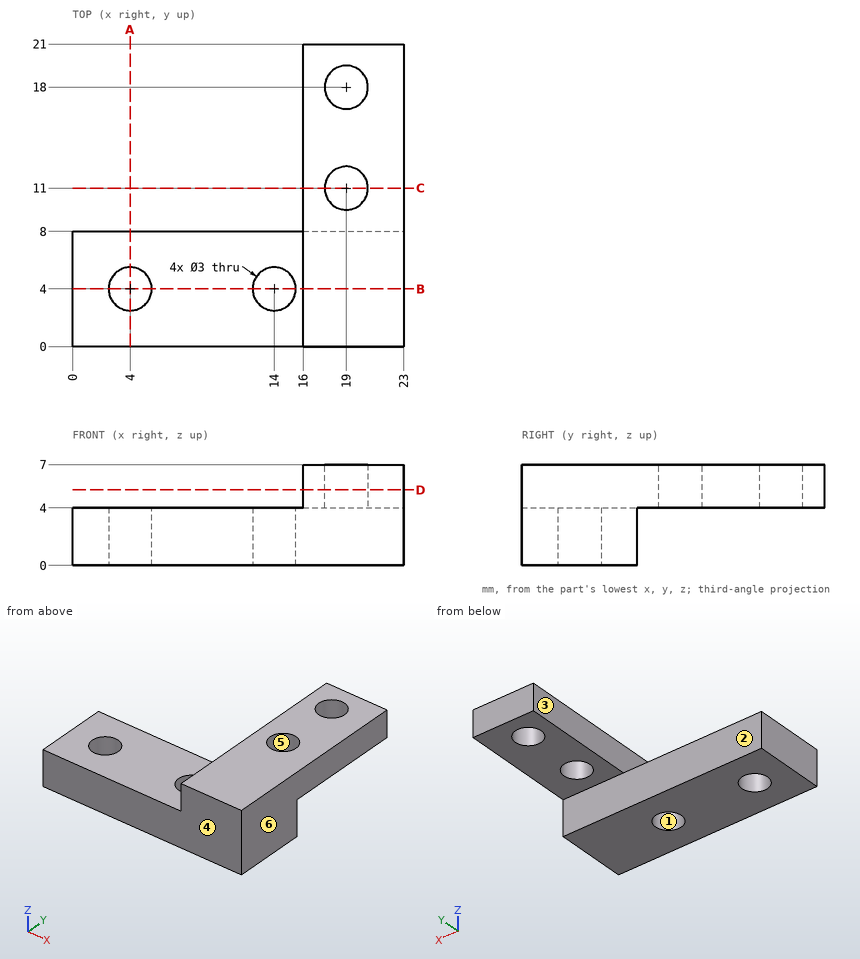
Geometry check sheet. Reference: drawing and pictorial views, mm from the part's lowest x, y, z. A direction names the side the tool comes from. Give positions to 0.01 mm unless a question says otherwise; leave off trailing zeros. Order: outer loops, then holes, each group sorted by start corner. A loop starts at its lowest first (then second) coordinate and runs counter-clockwise, first axis right, second up. Notation, with made-up numbers: (-2, -23) -> (2, -23) arc R34 ccw to (2, 8) -> close; hole circle Ø2 at (72.5, 29.5). An arc over 180 degrees is marked (long way). Use CSV: the item, a comma, the result in double quotes. Start each with the question number.
1) Sectioned sample at D-D, the plane z = 5.25. Record the boundary of the cut face in (x, y).
2) Sectioned sample at A-A, the plane x = 4. Record the boundary of the cut face in (y, z), plus the area to 3 significant figures.
3) Sectioned sample at C-C, the plane y = 11. Record the boundary of the cut face in (x, z), plus the area to 3 significant figures.
4) Go/stop test with flat-tipped pins: P1, Ø3, axis at y = 10, z = 4, coming from the -X side; P2, Ø1.2, axis at x = 14, z = 3, coming from the +Y side; P3, Ø3.5, axis at x = 21, y = 16, coming from the -Z side. Record where each tip stops, or that it passes through.
5) Material ranges on line 1 (Y direction, x = 19, z = 5.25); line 2 (Y direction, x = 4, z = 0.85); line 3 (X direction, y = 18.25, z = 4.5), recorded low to high. Write a range as from..to.
6) Sectioned sample at B-B, the plane y = 4. Record the boundary of the cut face in (x, z).
7) Set-up check for the marked faces 1, 2 and 3: record each of +Z, -Z, +X, -X, +Y, -Y from which the full face is reachable in a straight line by a thin tool's end or side.
8) Mould release check, pull along X, two halves, no side actions. Record for the marked faces 4, 5 and 6: released by +X, released by -X, zero draft, split by the parting line, or undercut.
Recorded:
1,outline,"(16, 0) -> (23, 0) -> (23, 21) -> (16, 21) -> close; hole circle Ø3 at (19, 11); hole circle Ø3 at (19, 18)"
2,outline,"(0, 0) -> (2.5, 0) -> (2.5, 4) -> (0, 4) -> close; (5.5, 0) -> (8, 0) -> (8, 4) -> (5.5, 4) -> close"
2,area,"20.0 mm2"
3,outline,"(16, 4) -> (17.5, 4) -> (17.5, 7) -> (16, 7) -> close; (20.5, 4) -> (23, 4) -> (23, 7) -> (20.5, 7) -> close"
3,area,"12.0 mm2"
4,P1,"x = 16"
4,P2,"y = 8"
4,P3,"z = 4"
5,line 1,"0..9.5, 12.5..16.5, 19.5..21"
5,line 2,"0..2.5, 5.5..8"
5,line 3,"16..17.52, 20.48..23"
6,outline,"(0, 0) -> (2.5, 0) -> (2.5, 4) -> (0, 4) -> close; (5.5, 0) -> (12.5, 0) -> (12.5, 4) -> (5.5, 4) -> close; (15.5, 0) -> (23, 0) -> (23, 7) -> (16, 7) -> (16, 4) -> (15.5, 4) -> close"
7,face 1,"+Z, -Z"
7,face 2,"-Z, +X, -X, +Y"
7,face 3,"+Z, -X, +Y, -Y"
8,face 4,"zero draft"
8,face 5,"undercut"
8,face 6,"released by +X"
